Work out the finished part from the listing and answer in its coordinate system (mm). A direction names the side the tool comes from. Round coordinates to 2 decimals unless told otherwise and drop trailing zeros. Order: outer loops, then holes, each group sorted by start corner. A loop starts at its lowest first (then second) coordinate and runs counter-clockwise, first axis right, second up. Notation, with made-up numbers: (-23, 3.5) - (27, 3.5) arc R10 ccw to (27, 8.5) - close; hole circle Ø6 at (37.25, -40). An arc over 180 degrees is marked (long way). Put each result on its own line as item: value.
```python
from build123d import *

# Parameters (mm, degrees)
SKETCH1_R          = 4
EXTRUDE1_DEPTH     = 16
CUT_EXTRUDE1_DEPTH = 2.5


with BuildPart() as part:
    # Sketch1 → Extrude1 (new body)
    with BuildSketch(Plane.XY):
        Circle(SKETCH1_R)
    extrude(amount=-EXTRUDE1_DEPTH)

    # Sketch2 → Revolve1 (revolve)
    with BuildSketch(Plane(origin=(0, 0, 0), x_dir=(0, 0, -1), z_dir=(1, 0, 0)), mode=Mode.PRIVATE) as revolve1_sk:
        with BuildLine():
            Line((0, 0), (0, 7))
            Line((0, 7), (-1, 7))
            ThreePointArc((-1, 7), (-3.404163056, 6.004163056), (-4.4, 3.6))
            Line((-4.4, 3.6), (-4.4, 0))
            Line((-4.4, 0), (0, 0))
        make_face()
    revolve(revolve1_sk.sketch.rotate(Axis((0, 0, 0), (0, 0, 1)), 90), axis=Axis((0, 0, 0), (0, 0, 1)))

    # Sketch3 → Cut-Extrude1 (cut)
    with BuildSketch(Plane.XY.offset(4.4)):
        Polygon((-1.443375673, 2.5), (-2.886751346, 0), (-1.443375673, -2.5), (1.443375673, -2.5), (2.886751346, 0), (1.443375673, 2.5), align=None)
    extrude(amount=-CUT_EXTRUDE1_DEPTH, mode=Mode.SUBTRACT)


solid = part.part
```
1) For a pull along X with two mould halves and no side action, classify faces 3 (the cylindrical face through (-0.867, -3.905, -7.888)), 4 (the flat face through (-2.175, -1.233, 3.168)), 5 (the flat face through (3, 3, 0)), 6 (the flat face through (2.155, -1.267, 3.168)) as pulls with the +X half, pulls with the -X half, needs draft (parallel to the pull), parting line crosses it, or undercut.
Findings below:
face 3: parting line crosses it
face 4: undercut
face 5: needs draft
face 6: undercut
2) For faces 1 (the flat face through (-2, 2, 4.4)), 2 (the flat face through (0, 2.5, 3)), determine the directions among +Z, -Z, +X, -X, +Y, -Y from which every point of the face is accessible in a straight line to the end or side of a thin tool.
Findings below:
face 1: +Z, +X, -X, +Y, -Y
face 2: +Z
3) Given pin 1 Ø8 at (x, y) = (-2.5, -3.5) entering from +Z; pin 2 Ø2 at (x, z) = (0.5, 3) entering from -Y; pin 3 Ø8 at (y, z) = (1.5, -5.5) entering from -X; pin 4 Ø3 at (x, z) = (3, -13) entering from -Y, each flat-ended and moving along its own axis, determine where each tip first touches the part or whether it passes through.
Findings below:
pin 1: stops at z = 4.4
pin 2: stops at y = -6.84
pin 3: stops at x = -4
pin 4: stops at y = -3.71
4) Straight lines are drawn through the part: L1, parallel to Y at x = 0.75, z = 2.5; L2, parallel to X at y = -6, z = 0.5; L3, parallel to Y at x = -3, z = -7.25. For each, find the intervals that lie inside material, in ascending order. Write a range as from..to.
Findings below:
L1: y = -6.61..-2.5, 2.5..6.61
L2: x = -3.61..3.61
L3: y = -2.65..2.65
5) A cutting plane is placed at A-A on x = 0. Write down the section's boundary in (y, z), then the cut area to 3 significant figures.
Findings below:
outline: (-7, 0) - (-4, 0) - (-4, -16) - (4, -16) - (4, 0) - (7, 0) - (7, 1) arc R3.4 ccw to (3.6, 4.4) - (2.5, 4.4) - (2.5, 1.9) - (-2.5, 1.9) - (-2.5, 4.4) - (-3.6, 4.4) arc R3.4 ccw to (-7, 1) - close
area: 172 mm2
6) A cutting plane is placed at B-B on z = -10.75. Write down the section's boundary in (x, y).
Findings below:
outline: circle Ø8 at (0, 0)
